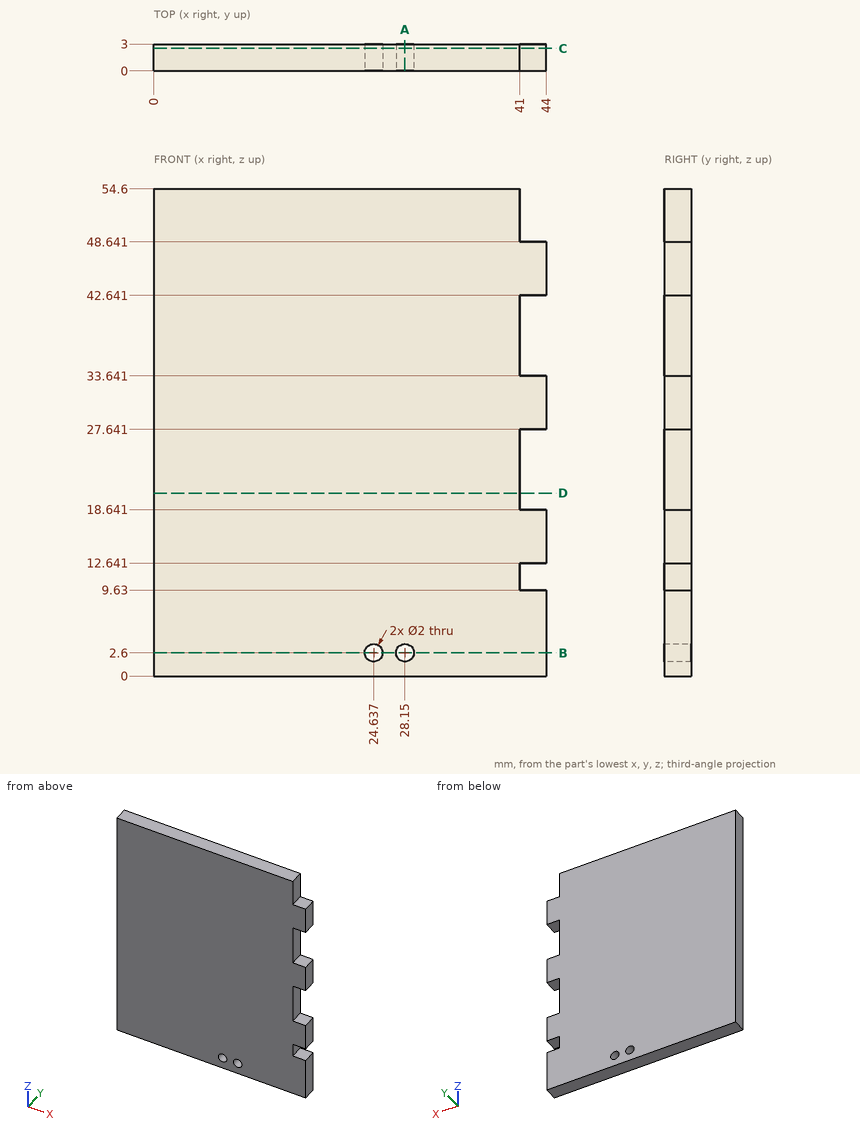
Study the drawing (mm; zero at the part's minimum x, y, z) and answer. Round coordinates to 2 decimals unless told otherwise and drop trailing zeros. Write each loop counter-clockwise with the first axis right and the second up, starting at its lowest first coordinate (ties: lowest second). Pieces come first, ordered by that corner, then holes.
1) Flat-ended cylindrical pins translate along their axes: P1, Ø1.5, axis at x = 42, y = 1.5, coming from the +Z side; P2, Ø0.9, axis at y = 1, z = 52, coming from the +X side; P3, Ø1.6, axis at x = 28.15, z = 2.6, coming from the -Y side. Find the tip coordinate at first contact, or state that the pin passes through.
2) A cutting plane is placed at B-B on z = 2.6. Determine the outline of the cut face in (x, y), and give its area (3 significant figures).
3) A cutting plane is placed at C-C on y = 2.5. Determine the outline of the cut face in (x, z).
4) A cutting plane is placed at D-D on z = 20.5. Determine the outline of the cut face in (x, y).
5) A cutting plane is placed at A-A on x = 28.15. Determine the outline of the cut face in (y, z), and give its area (3 significant figures).
6) Consider probe 1 along X at (y, z) = (1, 2.6); probe 2 along Z at (x, y) = (28, 1.6); probe 3 along Z at (x, y) = (42, 1.1). Determine where each line is inside the solid, lowest interval first.
Entries:
1. P1: stops at z = 48.64
1. P2: stops at x = 41
1. P3: passes through
2. outline: (0, 0) - (23.64, 0) - (23.64, 3) - (0, 3) - close; (25.64, 0) - (27.15, 0) - (27.15, 3) - (25.64, 3) - close; (29.15, 0) - (44, 0) - (44, 3) - (29.15, 3) - close
2. area: 120 mm2
3. outline: (0, 0) - (44, 0) - (44, 9.63) - (41, 9.63) - (41, 12.64) - (44, 12.64) - (44, 18.64) - (41, 18.64) - (41, 27.64) - (44, 27.64) - (44, 33.64) - (41, 33.64) - (41, 42.64) - (44, 42.64) - (44, 48.64) - (41, 48.64) - (41, 54.6) - (0, 54.6) - close; hole circle Ø2 at (24.64, 2.6); hole circle Ø2 at (28.15, 2.6)
4. outline: (0, 0) - (41, 0) - (41, 3) - (0, 3) - close
5. outline: (0, 0) - (3, 0) - (3, 1.6) - (0, 1.6) - close; (0, 3.6) - (3, 3.6) - (3, 54.6) - (0, 54.6) - close
5. area: 158 mm2
6. probe 1: x = 0 to 23.64, 25.64 to 27.15, 29.15 to 44
6. probe 2: z = 0 to 1.61, 3.59 to 54.6
6. probe 3: z = 0 to 9.63, 12.64 to 18.64, 27.64 to 33.64, 42.64 to 48.64
